from build123d import *

# Parameters (mm, degrees)
SKETCH_1_W          = 100
SKETCH_1_H          = 168
EXTRUDE_1_DEPTH     = 8
SKETCH_4_W          = 219.714234424
SKETCH_4_H          = 60.92406831
CUT_EXTRUDE_2_DEPTH = 8
SKETCH_5_W          = 131.187185814
SKETCH_5_H          = 64.749040209
CUT_EXTRUDE_3_DEPTH = 28
CUT_EXTRUDE_4_DEPTH = 198
SKETCH_7_W          = 88.901088493
SKETCH_7_H          = 24.075683618
CUT_EXTRUDE_5_DEPTH = 198
FILLET_2_R          = 5
CUT_EXTRUDE_6_DEPTH = 20
FILLET_3_R          = 10
EXTRUDE_2_DEPTH     = 8
CUT_EXTRUDE_7_DEPTH = 10
CHAMFER_1_SIZE      = 1


with BuildPart() as part:
    # 草图1 → 凸台-拉伸1 (new body)
    with BuildSketch(Plane.XY):
        Rectangle(SKETCH_1_W, SKETCH_1_H)
    extrude(amount=EXTRUDE_1_DEPTH)

    # 草图4 → 切除-拉伸2 (cut)
    with BuildSketch(Plane(origin=(-12.5, 0, 21.650635095), x_dir=(0, -1, 0), z_dir=(-0.499999999999998, 0, 0.8660254037844398))):
        with Locations((1.453456898, -25.633998951)):
            Rectangle(SKETCH_4_W, SKETCH_4_H)
    extrude(amount=CUT_EXTRUDE_2_DEPTH, mode=Mode.SUBTRACT)

    # 草图5 → 切除-拉伸3 (cut)
    with BuildSketch(Plane(origin=(0, 42, 42), x_dir=(-1, 0, 0), z_dir=(0, 0.7071067811865464, 0.7071067811865488))):
        with Locations((-5.06731619, -49.688146971)):
            Rectangle(SKETCH_5_W, SKETCH_5_H)
    extrude(amount=CUT_EXTRUDE_3_DEPTH, mode=Mode.SUBTRACT)

    # 草图6 → 切除-拉伸4 (cut)
    with BuildSketch(Plane.XZ.offset(84)):
        with BuildLine():
            Line((17.306736075, 0), (50, 0))
            Line((50, 0), (50, 8))
            Line((50, 8), (28.897086236, 8))
            ThreePointArc((28.897086236, 8), (23.578001039, 3.310243942), (17.306736075, 0))
        make_face()
    extrude(amount=-CUT_EXTRUDE_4_DEPTH, mode=Mode.SUBTRACT)

    # 草图7 → 切除-拉伸5 (cut)
    with BuildSketch(Plane(origin=(0, -59.535898385, -34.373066959), x_dir=(1, 0, 0), z_dir=(0, -0.866025403784438, -0.500000000000001))):
        with Locations((-5.418701979, 40.753668269)):
            Rectangle(SKETCH_7_W, SKETCH_7_H)
    extrude(amount=CUT_EXTRUDE_5_DEPTH, mode=Mode.SUBTRACT)

    # 圆角2
    # the kernel refuses this fillet: 5 mm, written as the material it takes off along each edge
    with BuildSketch(Plane(origin=(24.52361444, -79.381197846, 0), x_dir=(0, 1, 0), z_dir=(-1, 0, 0))) as fillet_2_piece_1:
        with BuildLine():
            CenterArc((FILLET_2_R * 0.57735026919, -FILLET_2_R), FILLET_2_R, 90, 60)
            Line((-FILLET_2_R * 0.288675134595, -FILLET_2_R * 0.5), (0, 0))
            Line((0, 0), (FILLET_2_R * 0.57735026919, 0))
        make_face()
    extrude(amount=74.392860666, mode=Mode.SUBTRACT)

    # 草图8 → 切除-拉伸6 (cut)
    with BuildSketch(Plane(origin=(0, 0, 0), x_dir=(-1, 0, 0), z_dir=(0, 0, -1))):
        Polygon((-60, 6), (-10, -44), (-10, -84), (0, -94), (-20, -94), (-60, -94), align=None)
    extrude(amount=-CUT_EXTRUDE_6_DEPTH, mode=Mode.SUBTRACT)

    # 圆角3
    fillet_3_edges = [part.edges().sort_by_distance(p)[0] for p in [
        (10, -44, 4),
    ]]
    fillet(fillet_3_edges, radius=FILLET_3_R)

    # 草图9 → 凸台-拉伸2 (add)
    with BuildSketch(Plane.XY.offset(8)):
        with BuildLine():
            ThreePointArc((-17.615836726, 56.159618943), (-16.143593539, 55.309618943), (-14.671350353, 56.159618943))
            Line((-14.671350353, 56.159618943), (-10.635451968, 63.15))
            ThreePointArc((-10.635451968, 63.15), (-10.635451968, 64.85), (-12.107695155, 65.7))
            Line((-12.107695155, 65.7), (-20.179491924, 65.7))
            ThreePointArc((-20.179491924, 65.7), (-21.651735111, 64.85), (-21.651735111, 63.15))
            Line((-21.651735111, 63.15), (-17.615836726, 56.159618943))
        make_face()
        with BuildLine():
            ThreePointArc((-17.615836726, 31.159618943), (-16.143593539, 30.309618943), (-14.671350353, 31.159618943))
            Line((-14.671350353, 31.159618943), (-10.635451968, 38.15))
            ThreePointArc((-10.635451968, 38.15), (-10.635451968, 39.85), (-12.107695155, 40.7))
            Line((-12.107695155, 40.7), (-20.179491924, 40.7))
            ThreePointArc((-20.179491924, 40.7), (-21.651735111, 39.85), (-21.651735111, 38.15))
            Line((-21.651735111, 38.15), (-17.615836726, 31.159618943))
        make_face()
        with BuildLine():
            ThreePointArc((-17.615836726, 6.159618943), (-16.143593539, 5.309618943), (-14.671350353, 6.159618943))
            Line((-14.671350353, 6.159618943), (-10.635451968, 13.15))
            ThreePointArc((-10.635451968, 13.15), (-10.635451968, 14.85), (-12.107695155, 15.7))
            Line((-12.107695155, 15.7), (-20.179491924, 15.7))
            ThreePointArc((-20.179491924, 15.7), (-21.651735111, 14.85), (-21.651735111, 13.15))
            Line((-21.651735111, 13.15), (-17.615836726, 6.159618943))
        make_face()
        with BuildLine():
            ThreePointArc((-17.615836726, -18.840381057), (-16.143593539, -19.690381057), (-14.671350353, -18.840381057))
            Line((-14.671350353, -18.840381057), (-10.635451968, -11.85))
            ThreePointArc((-10.635451968, -11.85), (-10.635451968, -10.15), (-12.107695155, -9.3))
            Line((-12.107695155, -9.3), (-20.179491924, -9.3))
            ThreePointArc((-20.179491924, -9.3), (-21.651735111, -10.15), (-21.651735111, -11.85))
            Line((-21.651735111, -11.85), (-17.615836726, -18.840381057))
        make_face()
        with BuildLine():
            ThreePointArc((-17.615836726, -43.840381057), (-16.143593539, -44.690381057), (-14.671350353, -43.840381057))
            Line((-14.671350353, -43.840381057), (-10.635451968, -36.85))
            ThreePointArc((-10.635451968, -36.85), (-10.635451968, -35.15), (-12.107695155, -34.3))
            Line((-12.107695155, -34.3), (-20.179491924, -34.3))
            ThreePointArc((-20.179491924, -34.3), (-21.651735111, -35.15), (-21.651735111, -36.85))
            Line((-21.651735111, -36.85), (-17.615836726, -43.840381057))
        make_face()
        with BuildLine():
            ThreePointArc((-10.635451968, -61.85), (-10.635451968, -60.15), (-12.107695155, -59.3))
            Line((-12.107695155, -59.3), (-20.179491924, -59.3))
            ThreePointArc((-20.179491924, -59.3), (-21.651735111, -60.15), (-21.651735111, -61.85))
            Line((-21.651735111, -61.85), (-17.615836726, -68.840381057))
            ThreePointArc((-17.615836726, -68.840381057), (-16.143593539, -69.690381057), (-14.671350353, -68.840381057))
            Line((-14.671350353, -68.840381057), (-10.635451968, -61.85))
        make_face()
    extrude(amount=EXTRUDE_2_DEPTH)

    # 草图10 → 切除-拉伸7 (cut)
    with BuildSketch(Plane(origin=(0, 0, 0), x_dir=(-1, 0, 0), z_dir=(0, 0, -1))):
        Polygon((-5.306736075, 84), (0.693263925, 78), (32, 78), (38, 84), align=None)
    extrude(amount=-CUT_EXTRUDE_7_DEPTH, mode=Mode.SUBTRACT)

    # 倒角1
    chamfer_1_edges = [part.edges().sort_by_distance(p)[0] for p in [
        (2.306736075, 81, 0),
        (-16.346631963, 78, 0),
        (-35, 81, 0),
    ]]
    chamfer(chamfer_1_edges, length=CHAMFER_1_SIZE)


solid = part.part
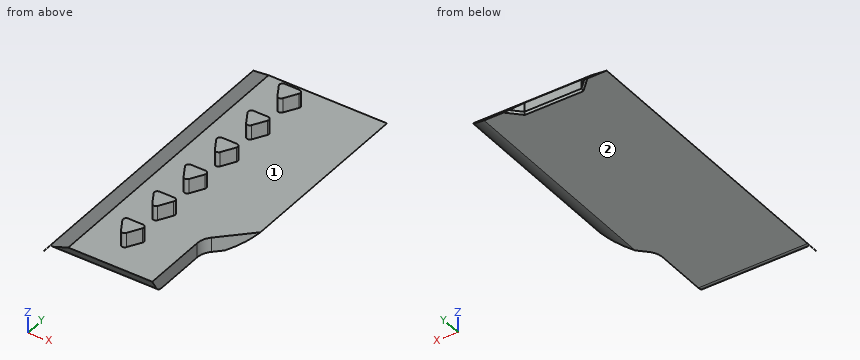
Can you work these out from the model? Positions are in its coordinate system, mm. Face numbers are marked on the shaded views. Give positions to 0.01 mm unless a question says otherwise; leave off trailing zeros. Loops run counter-clockwise (first coordinate to the right, second up) from the corner with the lowest first, then second, coordinate; pieces in that order, holes last. Notation, with made-up numbers: (75, 49.5) - (100, 49.5) arc R12 ccw to (100, 66.5) - close; hole circle Ø8 at (3.25, 55). An arc over 180 degrees is marked (long way). One line per item, written item: value.
(1) If we section it at B-B, the plane z = 13.5: State how many separate pieces and enclosed holes the cut face has, plus the area to 3 significant figures.
Verdict:
separate pieces: 6
enclosed holes: 0
area: 471 mm^2
(2) If we mould it in two halves opening along Z, with no side actions, what happens to the marked faces 1 and 2? For each: released by +Z, released by -Z, zero draft, split by the parting line, or undercut.
Verdict:
face 1: released by +Z
face 2: released by -Z
(3) If we section it at C-C, the plane y = 10.5: List the corners of the cut face in (x, z) for me, plus the area to 3 significant figures.
Verdict:
outline: (-50, 0) - (17.31, 0) arc R30 ccw to (28.9, 8) - (-12.17, 8) - (-12.17, 16) - (-20.12, 16) - (-20.12, 8) - (-36.14, 8) - close
area: 601 mm^2
(4) I'm going to push flat-ended pins straight in: pin 1 (1.5 mm diameter, centred on x = -22, z = 3, fed in from +Y); pin 2 (4 mm diameter, centred on x = -15, z = 14, fed in from +Y); pin 3 (5 mm diameter, centred on x = -17, z = 3, fed in from -Y). Where does each tip first touch, or does it pass through?
Verdict:
pin 1: y = 78
pin 2: y = 65.7
pin 3: y = -82.56
(5) If we section it at A-A, the plane x = -23.5: List the corners of the cut face in (y, z) for me, plus the area to 3 significant figures.
Verdict:
outline: (-84, 8) - (-80.82, 2.5) arc R5 ccw to (-76.49, 0) - (77, 0) - (78, 1) - (78, 6) - (76, 8) - close
area: 1,270 mm^2
(6) If we section it at D-D, the plane y = 73: List the corners of the cut face in (x, z) for me.
Verdict:
outline: (-50, 0) - (17.31, 0) arc R30 ccw to (28.9, 8) - (-36.14, 8) - close
(7) I need wall thicknesses on line 1 along Y through (x, z) = (-16.5, 9.25); line 2 along Z through (x, y) = (10, 64.5); line 3 along Y through (x, z) = (-17.5, 9). Which ranges of each line are inside material? Lowest first, please.
Verdict:
line 1: -69.65 to -59.3, -44.65 to -34.3, -19.65 to -9.3, 5.35 to 15.7, 30.35 to 40.7, 55.35 to 65.7
line 2: 0 to 8
line 3: -69.02 to -59.3, -44.02 to -34.3, -19.02 to -9.3, 5.98 to 15.7, 30.98 to 40.7, 55.98 to 65.7
